Geometry check sheet. Reference: the model listing, model coordinates, mm. A direction names the side the tool comes from. Give positions to 0.01 mm unless a question says otherwise; leave off trailing zeros. Order: outer loops, then holes, each group sorted by start corner. A loop starts at its lowest first (then second) coordinate and runs counter-clockwise, first axis right, second up. Notation, with made-up numbers: (71.25, 33) - (83.25, 33) arc R22 ccw to (83.25, 52) - close; hole circle Ø7 at (-22.5, 78). An arc over 180 degrees is marked (long way). Put each result on its own line as item: value. Start each with the question number.
```python
from build123d import *

# Parameters (mm, degrees)
SKETCH_1_R          = 7.5
EXTRUDE_4_DEPTH     = 7
SKETCH_4_W          = 40
SKETCH_4_H          = 2
EXTRUDE_5_DEPTH     = 7
SKETCH_5_W          = 16.420397205
SKETCH_5_H          = 7.153518057
CUT_EXTRUDE_1_DEPTH = 7
SKETCH_6_R          = 5.50001496
CUT_EXTRUDE_2_DEPTH = 7
SKETCH_7_W          = 11.00002992
SKETCH_7_H          = 1.975158718
CUT_EXTRUDE_3_DEPTH = 7
SKETCH_9_W          = 9.755837775
SKETCH_9_H          = 3.5
SKETCH_9_W_2        = 9.755837774
CUT_EXTRUDE_4_DEPTH = 7
SKETCH_10_W         = 1
SKETCH_10_H         = 3.5
EXTRUDE_6_DEPTH     = 2
SKETCH_11_W         = 1
SKETCH_11_H         = 3.5
EXTRUDE_7_DEPTH     = 2
SKETCH_12_R         = 5.944171322
EXTRUDE_8_DEPTH     = 7
SKETCH_13_W         = 14.038978355
SKETCH_13_H         = 4.452309985
CUT_EXTRUDE_5_DEPTH = 7
SKETCH_14_R         = 3.5
CUT_EXTRUDE_6_DEPTH = 7
SKETCH_15_W         = 7
SKETCH_15_H         = 1.975158718
CUT_EXTRUDE_7_DEPTH = 7


with BuildPart() as part:
    # 草图1 → 凸台-拉伸4 (new body)
    with BuildSketch(Plane(origin=(0, 0, 0), x_dir=(1, 0, 0), z_dir=(0, 1, 0))):
        with Locations(Location((0, 0, 0), (0, 0, 270))):
            Circle(SKETCH_1_R)
    extrude(amount=EXTRUDE_4_DEPTH)

    # 草图4 → 凸台-拉伸5 (add)
    with BuildSketch(Plane.XZ):
        with Locations((0.014666229, -0.975158718)):
            Rectangle(SKETCH_4_W, SKETCH_4_H)
    extrude(amount=-EXTRUDE_5_DEPTH)

    # 草图5 → 切除-拉伸1 (cut)
    with BuildSketch(Plane(origin=(0, 0, 0), x_dir=(-1, 0, 0), z_dir=(0, -1, 0))):
        with Locations((-0.974955135, 5.551917747)):
            Rectangle(SKETCH_5_W, SKETCH_5_H)
    extrude(amount=-CUT_EXTRUDE_1_DEPTH, mode=Mode.SUBTRACT)

    # 草图6 → 切除-拉伸2 (cut)
    with BuildSketch(Plane.XZ):
        Circle(SKETCH_6_R)
    extrude(amount=-CUT_EXTRUDE_2_DEPTH, mode=Mode.SUBTRACT)

    # 草图7 → 切除-拉伸3 (cut)
    with BuildSketch(Plane(origin=(0, 7, 0), x_dir=(1, 0, 0), z_dir=(0, 1, 0))):
        with Locations((0, 0.987579359)):
            Rectangle(SKETCH_7_W, SKETCH_7_H)
    extrude(amount=-CUT_EXTRUDE_3_DEPTH, mode=Mode.SUBTRACT)

    # 草图9 → 切除-拉伸4 (cut)
    with BuildSketch(Plane.XY.offset(0.024841282)):
        with Locations((-13.727128122, 3.659671281)):
            Rectangle(SKETCH_9_W, SKETCH_9_H)
        with Locations((13.812208225, 3.62574666)):
            Rectangle(SKETCH_9_W_2, SKETCH_9_H)
    extrude(amount=-CUT_EXTRUDE_4_DEPTH, mode=Mode.SUBTRACT)

    # 草图10 → 凸台-拉伸6 (add)
    with BuildSketch(Plane.XY.offset(0.024841282)):
        with Locations((18.190127112, 3.62574666)):
            Rectangle(SKETCH_10_W, SKETCH_10_H)
    extrude(amount=-EXTRUDE_6_DEPTH)

    # 草图11 → 凸台-拉伸7 (add)
    with BuildSketch(Plane.XY.offset(0.024841282)):
        with Locations((-18.10504701, 3.659671281)):
            Rectangle(SKETCH_11_W, SKETCH_11_H)
    extrude(amount=-EXTRUDE_7_DEPTH)

    # 草图12 → 凸台-拉伸8 (add)
    with BuildSketch(Plane(origin=(0, 0, 0), x_dir=(-1, 0, 0), z_dir=(0, -1, 0))):
        Circle(SKETCH_12_R)
    extrude(amount=-EXTRUDE_8_DEPTH)

    # 草图13 → 切除-拉伸5 (cut)
    with BuildSketch(Plane(origin=(0, 0, 0), x_dir=(-1, 0, 0), z_dir=(0, -1, 0))):
        with Locations((-1.413071361, 4.201313711)):
            Rectangle(SKETCH_13_W, SKETCH_13_H)
    extrude(amount=-CUT_EXTRUDE_5_DEPTH, mode=Mode.SUBTRACT)

    # 草图14 → 切除-拉伸6 (cut)
    with BuildSketch(Plane.XZ):
        Circle(SKETCH_14_R)
    extrude(amount=-CUT_EXTRUDE_6_DEPTH, mode=Mode.SUBTRACT)

    # 草图15 → 切除-拉伸7 (cut)
    with BuildSketch(Plane.XZ):
        with Locations((0, -0.987579359)):
            Rectangle(SKETCH_15_W, SKETCH_15_H)
    extrude(amount=-CUT_EXTRUDE_7_DEPTH, mode=Mode.SUBTRACT)


solid = part.part
```
Item 1: Set-up check for faces 4 (the face through (14, 6, 0.025)), 5 (the face through (17.69, 4, -1)), 6 (the face through (3.5, 3, -1)), 7 (the face through (-14, 1, 0.025)): record each of +Z, -Z, +X, -X, +Y, -Y from which the full face is reachable in a straight line by a thin tool's end or side.
Item 2: Release check for a two-part mould opening along X. For faces 1 (the face through (-0.16, 3.45, 7.5)), 2 (the face through (-13, 5.41, -1)), 3 (the face through (12, 6, -1.975)) record: +X half, -X half, draft (parallel to the pull), parting line (faces both ways), or undercut.
Item 3: Cross-section at B-B (x = -11.5). Enter the section's corners in (y, z), and give its area (3 significant figures).
Item 4: Cross-section at C-C (z = 1.5). Enter the section's corners in (x, y).
Item 5: Cross-section at A-A (y = 3.5). Enter the section's corners in (x, z).
Item 6: Cross-section at D-D (y = 5.75). Enter the section's corners in (x, z).
Item 7: Gauge pin test, flat ends, axial feed: pin 1 Ø1 at (x, z) = (-2, 3) entering from -Y; pin 2 Ø1.5 at (x, y) = (-14.5, 3.5) entering from -Z; pin 3 Ø2 at (x, y) = (-15.5, 5) entering from +Z; pin 4 Ø1.5 at (x, y) = (-4, 1.5) entering from +Z. Record the tip position at first contact, or that the pin passes through.
Item 8: Thickness scan on line 1 along Y through (x, z) = (-16, -1.5); line 2 along Z through (x, y) = (18, 4.5); line 3 along X through (y, z) = (1, -1). Record the ranges inside material, lowest first.
Recorded:
1. face 4: +Z, +X, +Y, -Y
1. face 5: +Z, -Z
1. face 6: -Z, +Y, -Y
1. face 7: +Z, -X, +Y, -Y
2. face 1: parting line
2. face 2: undercut
2. face 3: draft
3. outline: (0, -1.98) - (1.91, -1.98) - (1.91, 0.02) - (0, 0.02) - close; (5.41, -1.98) - (7, -1.98) - (7, 0.02) - (5.41, 0.02) - close
3. area: 7.00 mm^2
4. outline: (-7.35, 0) - (-3.16, 0) - (-3.16, 7) - (-7.35, 7) - close; (3.16, 0) - (7.35, 0) - (7.35, 7) - (3.16, 7) - close
5. outline: (-19.99, -1.98) - (-17.61, -1.98) - (-17.61, 0.02) - (-19.99, 0.02) - close; (-8.85, -1.98) - (-3.5, -1.98) - (-3.5, 0) arc R3.5 cw to (3.5, 0) - (3.5, -1.98) - (8.93, -1.98) - (8.93, 0.02) - (7.5, 0.02) arc R7.5 ccw to (-7.5, 0.02) - (-8.85, 0.02) - close; (17.69, -1.98) - (20.01, -1.98) - (20.01, 0.02) - (17.69, 0.02) - close
6. outline: (-19.99, -1.98) - (-3.5, -1.98) - (-3.5, 0) arc R3.5 cw to (3.5, 0) - (3.5, -1.98) - (20.01, -1.98) - (20.01, 0.02) - (7.5, 0.02) arc R7.5 ccw to (-7.5, 0.02) - (-19.99, 0.02) - close
7. pin 1: stops at y = 0
7. pin 2: passes through
7. pin 3: stops at z = 0.02
7. pin 4: stops at z = 6.76
8. line 1: y = 0 to 1.91, 5.41 to 7
8. line 2: z = -1.98 to 0.02
8. line 3: x = -19.99 to -3.5, 3.5 to 20.01
